Could you check a few things on this model? Use its own coordinates, in mm. Face numbers are marked on the shaded views. A direction names the side the tool comes from. Coordinates: 2 decimals unless noted, no trailing zeros. Order: outer loops, then holes, each group sorted by start corner. A loop starts at its lowest first (then second) coordinate and runs counter-clockwise, first axis right, second up. Notation, with made-up numbers: (68.25, 57) -> (92.25, 57) arc R22 cw to (92.25, 92) -> close; hole circle Ø7 at (-23, -1.5). An arc over 180 degrees is marked (long way). Put each result on its own line as item: value. Start each with the question number.
Q1. Please list where these lines run through material, in increasing order: line 1 along Y through (x, z) = (-13, 2); line 2 along Z through (x, y) = (24, -5.5); line 3 along Z through (x, y) = (11, -5.5).
Q2. If we section it at B-B (z = 2.5): Count the separate pieces of the cut face and the enclosed holes in it, and give its area (3 significant figures).
Q3. If we section it at A-A (z = 6): Please give me the cut outline in (x, y).
Q4. For the marked faces 1, 2, 3, 4 and 5, which set-ups out of +Z, -Z, +X, -X, +Y, -Y let a thin tool reach every point of the face, with its end or its side?
Q5. Will these pins go through, and if not, where does the flat tip stop? pin 1 (2.5 mm diameter, centred on x = 26.21, y = -14.63, fed in from +Z); pin 2 (1.6 mm diameter, centred on y = -8.5, z = 3, fed in from +X); pin 3 (1.7 mm diameter, centred on x = 26.5, y = -14, fed in from +Z); pin 4 (6 mm diameter, centred on x = 7.5, y = -7.5, fed in from -Z).
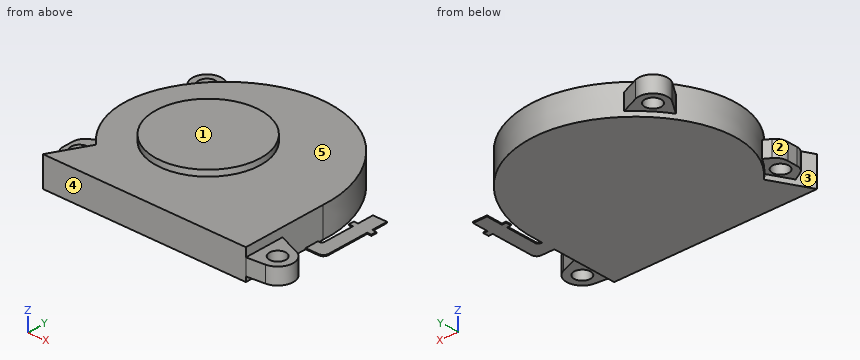
from build123d import *

# Parameters (mm, degrees)
SKIZZE1_R                       = 12.15
SKIZZE1_R_2                     = 9.65
AUFSATZ_LINEAR_AUSTRAGEN1_DEPTH = 5.5
SKIZZE1_3_R                     = 9.65
AUFSATZ_LINEAR_AUSTRAGEN2_DEPTH = 6.6
AUFSATZ_LINEAR_START            = 0.9
SKIZZE1_5_R                     = 1.5
AUFSATZ_LINEAR_AUSTRAGEN3_DEPTH = 3
AUFSATZ_LINEAR_AUSTRAGEN4_DEPTH = 0.2


with BuildPart() as part:
    # Skizze1 → Aufsatz-Linear austragen1 (new body)
    # profile 1 of 2: a face of its own
    with BuildSketch(Plane.XY):
        with BuildLine():
            Line((23.22989124, -17.8), (23.22989124, -2.247542747))
            add(Edge.make_bspline(
                [(23.22989124, -2.247542747), (23.570505731, 5.01843493), (17.435920317, 16.509432663), (2.315543688, 19.773891452), (-13.917413027, 13.221960429), (-19.306383662, -2.33852969), (-10.663184769, -11.056444767)],
                knots=[0, 0, 0, 0, 0.303535836, 0.457029394, 0.601755461, 1, 1, 1, 1], degree=3))
            Line((-10.663184769, -11.056444767), (-14.24879669, -17.8))
            Line((-14.24879669, -17.8), (23.22989124, -17.8))
        make_face()
        Circle(SKIZZE1_R, mode=Mode.SUBTRACT)
    # profile 2 of 2: a face of its own
    with BuildSketch(Plane.XY):
        Circle(SKIZZE1_R)
        Circle(SKIZZE1_R_2, mode=Mode.SUBTRACT)
    extrude(amount=AUFSATZ_LINEAR_AUSTRAGEN1_DEPTH)

    # Skizze1_3 → Aufsatz-Linear austragen2 (add)
    with BuildSketch(Plane.XY):
        Circle(SKIZZE1_3_R)
    extrude(amount=AUFSATZ_LINEAR_AUSTRAGEN2_DEPTH)

    # Skizze1_5 → Aufsatz-Linear austragen3 (add)
    # profile 1 of 3: a face of its own
    with BuildSketch(Plane.XY.offset(AUFSATZ_LINEAR_START)):
        with BuildLine():
            add(Edge.make_bspline(
                [(-8.069037879, 14.42388259), (-9.937212437, 12.945618154), (-11.560246269, 11.14536638), (-12.81225318, 9.143669748)],
                knots=[0.61161883, 0.61161883, 0.61161883, 0.61161883, 0.708712293, 0.708712293, 0.708712293, 0.708712293], degree=3))
            Line((-8.069037879, 14.42388259), (-11.430379202, 15.82207236))
            ThreePointArc((-11.430379202, 15.82207236), (-14.493909546, 15.059392032), (-14.653056668, 11.90636624))
            Line((-14.653056668, 11.90636624), (-12.81225318, 9.143669748))
        make_face()
        with Locations((-12.448019378, 13.375597605)):
            Circle(SKIZZE1_5_R, mode=Mode.SUBTRACT)
    # profile 2 of 3: a face of its own
    with BuildSketch(Plane.XY.offset(AUFSATZ_LINEAR_START)):
        with BuildLine():
            Line((23.22989124, -10.418487336), (23.22989124, -17.8))
            Line((23.22989124, -17.8), (26.500672864, -17.459737855))
            ThreePointArc((26.500672864, -17.459737855), (29.026515796, -15.008489952), (27.237700891, -11.977212988))
            Line((27.237700891, -11.977212988), (23.22989124, -10.418487336))
        make_face()
        with Locations((26.206225463, -14.629352042)):
            Circle(SKIZZE1_5_R, mode=Mode.SUBTRACT)
    # profile 3 of 3: a face of its own
    with BuildSketch(Plane.XY.offset(AUFSATZ_LINEAR_START)):
        with BuildLine():
            Line((-14.434796379, -14.178445133), (-12.800547832, -15.076240045))
            Line((-12.800547832, -15.076240045), (-10.663184769, -11.056444767))
            add(Edge.make_bspline(
                [(-13.215759107, -7.863797122), (-12.531518629, -8.956537973), (-11.685451286, -10.025341262), (-10.663184769, -11.056444767)],
                knots=[0.952897988, 0.952897988, 0.952897988, 0.952897988, 1, 1, 1, 1], degree=3))
            Line((-13.215759107, -7.863797122), (-14.363260793, -8.582327138))
            ThreePointArc((-14.363260793, -8.582327138), (-15.186624929, -9.485521456), (-15.423283617, -10.684554877))
            Line((-15.423283617, -10.684554877), (-15.423283617, -12.507578786))
            ThreePointArc((-15.423283617, -12.507578786), (-15.157656262, -13.478261712), (-14.434796379, -14.178445133))
        make_face()
        with Locations((-13.17621437, -11.618483702)):
            Circle(SKIZZE1_5_R, mode=Mode.SUBTRACT)
    extrude(amount=AUFSATZ_LINEAR_AUSTRAGEN3_DEPTH)

    # Skizze1_6 → Aufsatz-Linear austragen4 (add)
    with BuildSketch(Plane.XY):
        with BuildLine():
            Line((23.22989124, -3.252529258), (23.22989124, -5.733420738))
            Line((23.22989124, -5.733420738), (25.665000561, -5.733420738))
            ThreePointArc((25.665000561, -5.733420738), (26.331877002, -5.457191471), (26.608106269, -4.79031503))
            Line((26.608106269, -4.79031503), (26.608106269, 3.027890879))
            Line((26.608106269, 3.027890879), (27.408106269, 3.027890879))
            Line((27.408106269, 3.027890879), (27.408106269, 4.027890879))
            Line((27.408106269, 4.027890879), (26.608106269, 4.027890879))
            Line((26.608106269, 4.027890879), (26.608106269, 7.027890879))
            Line((26.608106269, 7.027890879), (24.008106269, 7.027890879))
            Line((24.008106269, 7.027890879), (24.008106269, 4.027890879))
            Line((24.008106269, 4.027890879), (23.208106269, 4.027890879))
            Line((23.208106269, 4.027890879), (23.208106269, 3.027890879))
            Line((23.208106269, 3.027890879), (24.008106269, 3.027890879))
            Line((24.008106269, 3.027890879), (24.008106269, -2.725622817))
            ThreePointArc((24.008106269, -2.725622817), (23.853778945, -3.098201935), (23.481199827, -3.252529258))
            Line((23.481199827, -3.252529258), (23.22989124, -3.252529258))
        make_face()
    extrude(amount=AUFSATZ_LINEAR_AUSTRAGEN4_DEPTH)


solid = part.part
The answers:
1. line 1: -17.8 to -15.45, -14.97 to -13.11, -10.13 to 8.84, 9.43 to 11.98, 14.77 to 15.97
1. line 2: 0 to 0.2
1. line 3: 0 to 5.5
2. separate pieces: 1
2. enclosed holes: 3
2. area: 1,270 mm^2
3. outline: circle Ø19.3 at (0, 0)
4. face 1: +Z, +X, -X, +Y, -Y
4. face 2: +Z, -Z, -X
4. face 3: -X
4. face 4: +Z, -Z, +X, -X, -Y
4. face 5: +Z
5. pin 1: through
5. pin 2: x = 23.23
5. pin 3: z = 3.9
5. pin 4: z = 0
